from build123d import *

# Parameters (mm, degrees)
SKETCH2_W           = 200
SKETCH2_H           = 100
BOSS_EXTRUDE2_DEPTH = 20


with BuildPart() as part:
    # Sketch2 → Boss-Extrude2 (new body)
    with BuildSketch(Plane(origin=(0, 0, 0), x_dir=(1, 0, 0), z_dir=(0, 1, 0))):
        Rectangle(SKETCH2_W, SKETCH2_H)
        with BuildLine():
            Line((-39.130434783, 15), (39.130434783, 15))
            ThreePointArc((39.130434783, 15), (54.130434783, 0), (39.130434783, -15))
            Line((39.130434783, -15), (-39.130434783, -15))
            ThreePointArc((-39.130434783, -15), (-54.130434783, 0), (-39.130434783, 15))
        make_face(mode=Mode.SUBTRACT)
    extrude(amount=BOSS_EXTRUDE2_DEPTH)


solid = part.part
For this review, take the finished solid that the model builds, in its own axes (mm). A direction names the side the tool comes from. Give positions to 0.01 mm unless a question says otherwise; leave off trailing zeros. Loops run counter-clockwise (first coordinate to the right, second up) from the corner with the lowest first, then second, coordinate; pieces in that order, holes last. Notation, with made-up numbers: (85, -35) - (111, -35) arc R22 ccw to (111, -2) - close; hole circle Ø9 at (-39, 87). An arc over 180 degrees is marked (long way). Write each question's results on one line, items separated by ' | '.
(1) For faces 1 (the flat face through (-1, 0, -23)), 2 (the cylindrical face through (54.127, 9.86, -0.33)), list the 3-axis set-ups (+Z, -Z, +X, -X, +Y, -Y) from which the entire face can be reached by the end or side of a thin tool; tool diameter is ignored.
Conclusion:
face 1: +Z, -Z, +X, -X, -Y | face 2: +Y, -Y
(2) Draft analysis for pull direction X (two halves, no side actions). For faces 3 (the flat face through (-1, 10, -15)), 4 (the flat face through (1, 10, 15)), 5 (the flat face through (-1, 10, -50)), 6 (the flat face through (100, 10, 1)), state which applies: +X half, -X half, draft (parallel to the pull), parting line (faces both ways), or undercut.
Conclusion:
face 3: undercut | face 4: undercut | face 5: draft | face 6: +X half
(3) Take a section at B-B (z = 0). Give the boundary of the cut face in (x, y).
Conclusion:
outline: (-100, 0) - (-54.13, 0) - (-54.13, 20) - (-100, 20) - close; (54.13, 0) - (100, 0) - (100, 20) - (54.13, 20) - close
(4) Take a section at C-C (y = 14). Give the boundary of the cut face in (x, z), then the cut area to 3 significant figures.
Conclusion:
outline: (-100, -50) - (100, -50) - (100, 50) - (-100, 50) - close; hole (-39.13, -15) - (39.13, -15) arc R15 ccw to (39.13, 15) - (-39.13, 15) arc R15 ccw to start | area: 16,900 mm^2
(5) Take a section at A-A (x = -7). Give the boundary of the cut face in (y, z), then the cut area to 3 significant figures.
Conclusion:
outline: (0, -50) - (20, -50) - (20, -15) - (0, -15) - close; (0, 15) - (20, 15) - (20, 50) - (0, 50) - close | area: 1,400 mm^2
(6) For line 1 along Z through (x, y) = (23, 18.5); line 2 along Z through (x, y) = (45, 1.25); line 3 along X through (y, z) = (14, -6), list the stretches that pass through material, from the lowest coordinate up.
Conclusion:
line 1: -50 to -15, 15 to 50 | line 2: -50 to -13.8, 13.8 to 50 | line 3: -100 to -52.88, 52.88 to 100
